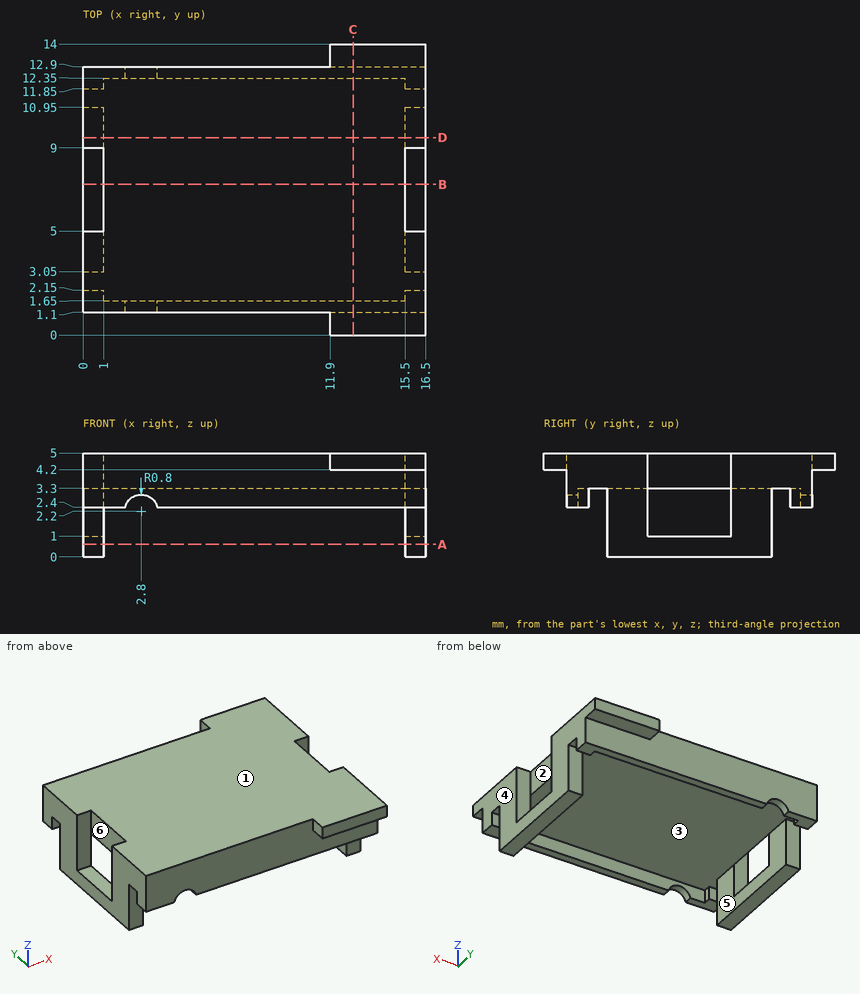
Input: dimensioned drawing with shaded views. Units: mm. Origin: part minimum x, y, z. A direction names the side the tool comes from. Coordinates: 2 decimals unless noted, no trailing zeros. Loops run counter-clockwise (first coordinate to the right, second up) from the corner with the lowest first, then second, coordinate; pieces in that order, holes last. Notation, with made-up numbers: (55, -24.75) -> (85, -24.75) arc R24 cw to (85, 2.25) -> close; hole circle Ø6 at (-33, 44.5). An arc over 180 degrees is marked (long way). Use a Markdown table: item, result. Add a question column.
(1) Pin query (flat end, axial travel): pin 1 Ø0.5 at (x, z) = (16, 3) entering from -Y; pin 2 Ø3 at (x, z) = (11, 4) entering from -Y; pin 3 Ø0.7 at (x, z) = (16, 2.5) entering from +Y; pin 4 Ø1.4 at (y, z) = (6, 4) entering from -X. Return the tip coordinate at first contact, or that it passes through.
(2) Mould query, pull axis Y, two halves, no side actions, for the marked faces 1, 2 and 3. Classes: pulls with the +Y half, pulls with the -Y half, needs draft (parallel to the pull), parting line crosses it, or undercut.
(3) Access query for the marked faces 4, 5 and 6. Directions: +Z, -Z, +X, -X, +Y, -Y. A direction counts if a zero-diameter tool reaches every point of the face in a straight line with its end or side. Return the directions, or none.
(4) Line query: line 1 along X through (y, z) = (10.25, 0.5); line 2 along Y through (x, z) = (10, 3.25); line 3 along Z through (x, y) = (9, 7.75). Output: solid intervals per line, ascending.
(5) Section query D-D, the plane y = 9.5. Return loops of the section in (x, z), plus the area to 4 significant figures.
(6) Section query A-A, the plane z = 0.6. Return loops of the section in (x, y), plus the area to 3 significant figures.
(7) Section query B-B, the plane y = 7.25. Return loops of the section in (x, z).
(8) Section query C-C, the plane x = 13. Return loops of the section in (y, z).
Answer:
| question | item | result |
|---|---|---|
| 1 | pin 1 | stops at y = 1.1 |
| 1 | pin 2 | stops at y = 0 |
| 1 | pin 3 | stops at y = 12.9 |
| 1 | pin 4 | stops at x = 1 |
| 2 | face 1 | needs draft |
| 2 | face 2 | undercut |
| 2 | face 3 | undercut |
| 3 | face 4 | +Z, -Z, +X, +Y, -Y |
| 3 | face 5 | -Z |
| 3 | face 6 | +Z, -X |
| 4 | line 1 | x = 0 to 1, 15.5 to 16.5 |
| 4 | line 2 | y = 1.1 to 1.65, 12.35 to 12.9 |
| 4 | line 3 | z = 3.3 to 5 |
| 5 | outline | (0, 0) -> (1, 0) -> (1, 3.3) -> (15.5, 3.3) -> (15.5, 0) -> (16.5, 0) -> (16.5, 5) -> (0, 5) -> close |
| 5 | area | 34.65 mm^2 |
| 6 | outline | (0, 3.05) -> (1, 3.05) -> (1, 10.95) -> (0, 10.95) -> close; (15.5, 3.05) -> (16.5, 3.05) -> (16.5, 10.95) -> (15.5, 10.95) -> close |
| 6 | area | 15.8 mm^2 |
| 7 | outline | (0, 0) -> (1, 0) -> (1, 1) -> (0, 1) -> close; (1, 3.3) -> (15.5, 3.3) -> (15.5, 5) -> (1, 5) -> close; (15.5, 0) -> (16.5, 0) -> (16.5, 1) -> (15.5, 1) -> close |
| 8 | outline | (0, 4.2) -> (1.1, 4.2) -> (1.1, 2.4) -> (1.65, 2.4) -> (1.65, 3.3) -> (12.35, 3.3) -> (12.35, 2.4) -> (12.9, 2.4) -> (12.9, 4.2) -> (14, 4.2) -> (14, 5) -> (0, 5) -> close |
